```python
from build123d import *

# Parameters (mm, degrees)
PAD_DEPTH     = 2
SKETCH001_R   = 2
PAD001_DEPTH  = 4
PAD002_DEPTH  = 5
SKETCH003_W   = 60
SKETCH003_H   = 16
SKETCH003_W_2 = 25
SKETCH003_H_2 = 42
POCKET_DEPTH  = 2


with BuildPart() as part:
    # Sketch → Pad (new body)
    with BuildSketch(Plane.XY):
        with BuildLine():
            Line((5.000023, 0), (114.999975, 0))
            ThreePointArc((114.999975, 0), (118.535523, 1.464455), (120, 4.999992))
            Line((120, 4.999992), (120, 51.000008))
            ThreePointArc((120, 51.000008), (118.535523, 54.535545), (114.999975, 56))
            Line((5.000023, 56), (114.999975, 56))
            ThreePointArc((5.000023, 56), (1.464477, 54.535545), (0, 51.000008))
            Line((0, 51.000008), (0, 4.999992))
            ThreePointArc((0, 4.999992), (1.464477, 1.464455), (5.000023, 0))
        make_face()
    extrude(amount=PAD_DEPTH)

    # Sketch001 → Pad001 (new body)
    with BuildSketch(Plane.XY.offset(2)):
        with Locations((10, 46)):
            Circle(SKETCH001_R)
        with Locations((38, 46)):
            Circle(SKETCH001_R)
        with Locations((10, 10)):
            Circle(SKETCH001_R)
        with Locations((38, 10)):
            Circle(SKETCH001_R)
    extrude(amount=PAD001_DEPTH)

    # Sketch002 → Pad002 (new body)
    with BuildSketch(Plane.XY.offset(2)):
        Polygon((55, 43.5), (55, 49.5), (61, 49.5), (61, 47.5), (57, 47.5), (57, 43.5), align=None)
        Polygon((72.5, 47.5), (72.5, 49.5), (78.5, 49.5), (78.5, 43.5), (76.5, 43.5), (76.5, 47.5), align=None)
        Polygon((55, 12.5), (57, 12.5), (57, 8.5), (61, 8.5), (61, 6.5), (55, 6.5), align=None)
        Polygon((76.5, 12.5), (78.5, 12.5), (78.5, 6.5), (72.5, 6.5), (72.5, 8.5), (76.5, 8.5), align=None)
    extrude(amount=PAD002_DEPTH)

    # Sketch003 → Pocket (cut)
    with BuildSketch(Plane.XY.offset(2)):
        with Locations((45, 28)):
            Rectangle(SKETCH003_W, SKETCH003_H)
        with Locations((100.5, 27)):
            Rectangle(SKETCH003_W_2, SKETCH003_H_2)
    extrude(amount=-POCKET_DEPTH, mode=Mode.SUBTRACT)


solid = part.part
```
Here's how the part is built. I have some questions about the finished solid (model axes, mm). A direction names the side the tool comes from. Round coordinates to 2 decimals unless told otherwise and drop trailing zeros. Order: outer loops, then holes, each group sorted by start corner. A loop starts at its lowest first (then second) coordinate and runs counter-clockwise, first axis right, second up. Notation, with made-up numbers: (-9.75, 11) -> (19.25, 11) arc R21 cw to (19.25, 39) -> close; hole circle Ø1 at (-25, -8.75). An arc over 180 degrees is marked (long way). Use a Markdown table: item, result. Add a question column.
(1) For faces 4 (the face through (57, 11, 4)), 5 (the face through (56, 12.5, 4)), 6 (the face through (75, 49.5, 4)), 7 (the face through (58, 6.5, 4)), 8 (the face through (61, 49, 4)), which set-ups out of +Z, -Z, +X, -X, +Y, -Y let a thin tool reach every point of the face, with its end or its side?
(2) Suppose I cut it at A-A, the plane x = 93. Please give me the cut outline in (y, z).
(3) For pin 1 Ø2.5 at (y, z) = (46.5, 5) entering from -X; pin 2 Ø1.2 at (x, y) = (38, 45.5) entering from +Z; pin 3 Ø0.6 at (x, z) = (77.5, 5.5) entering from +Y; pin 4 Ø1.5 at (x, z) = (84, 4.5) entering from +Y, each with a flat end and sliding along its axis, tell me the tip position at first contact or that it passes through.
(4) If we mould it in two halves opening along X, with no side actions, what happens to faces 1 (the face through (2, 55, 1)), 2 (the face through (120, 28, 1)), 3 (the face through (57, 46, 4))? For each: released by +X, released by -X, zero draft, split by the parting line, or undercut.
(5) Suppose I cut it at C-C, the plane y = 10. Please give me the cut outline in (x, z).
(6) I need wall thicknesses on line 1 along X through (y, z) = (33, 0.75); line 2 along X through (y, z) = (48, 6.5); line 3 along Y through (x, z) = (18, 1.5). Which ranges of each line are inside material? Lowest first, please.
(7) Suppose I cut it at D-D, the plane y = 25. Please give me the cut outline in (x, z), and give its area (3 significant figures).
(8) Suppose I cut it at B-B, the plane z = 3.5. Please give me the cut outline in (x, y), and give its area (3 significant figures).
Verdict:
| question | item | result |
|---|---|---|
| 1 | face 4 | +Z |
| 1 | face 5 | +Z, +X, -X |
| 1 | face 6 | +Z, +X, -X, +Y |
| 1 | face 7 | +Z, +X, -X, -Y |
| 1 | face 8 | +Z, +Y, -Y |
| 2 | outline | (0, 0) -> (6, 0) -> (6, 2) -> (0, 2) -> close; (48, 0) -> (56, 0) -> (56, 2) -> (48, 2) -> close |
| 3 | pin 1 | x = 8 |
| 3 | pin 2 | z = 6 |
| 3 | pin 3 | y = 49.5 |
| 3 | pin 4 | through |
| 4 | face 1 | released by -X |
| 4 | face 2 | released by +X |
| 4 | face 3 | undercut |
| 5 | outline | (0, 0) -> (88, 0) -> (88, 2) -> (78.5, 2) -> (78.5, 7) -> (76.5, 7) -> (76.5, 2) -> (57, 2) -> (57, 7) -> (55, 7) -> (55, 2) -> (40, 2) -> (40, 6) -> (36, 6) -> (36, 2) -> (12, 2) -> (12, 6) -> (8, 6) -> (8, 2) -> (0, 2) -> close; (113, 0) -> (120, 0) -> (120, 2) -> (113, 2) -> close |
| 6 | line 1 | 0 to 15, 75 to 88, 113 to 120 |
| 6 | line 2 | 55 to 61, 72.5 to 78.5 |
| 6 | line 3 | 0 to 20, 36 to 56 |
| 7 | outline | (0, 0) -> (15, 0) -> (15, 2) -> (0, 2) -> close; (75, 0) -> (88, 0) -> (88, 2) -> (75, 2) -> close; (113, 0) -> (120, 0) -> (120, 2) -> (113, 2) -> close |
| 7 | area | 70.0 mm2 |
| 8 | outline | circle Ø4 at (10, 10); circle Ø4 at (10, 46); circle Ø4 at (38, 10); circle Ø4 at (38, 46); (55, 6.5) -> (61, 6.5) -> (61, 8.5) -> (57, 8.5) -> (57, 12.5) -> (55, 12.5) -> close; (55, 43.5) -> (57, 43.5) -> (57, 47.5) -> (61, 47.5) -> (61, 49.5) -> (55, 49.5) -> close; (72.5, 6.5) -> (78.5, 6.5) -> (78.5, 12.5) -> (76.5, 12.5) -> (76.5, 8.5) -> (72.5, 8.5) -> close; (72.5, 47.5) -> (76.5, 47.5) -> (76.5, 43.5) -> (78.5, 43.5) -> (78.5, 49.5) -> (72.5, 49.5) -> close |
| 8 | area | 130 mm2 |
